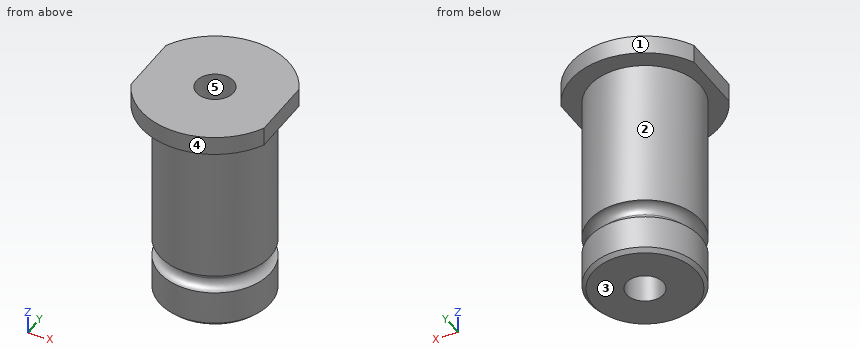
from build123d import *

# Parameters (mm, degrees)
F1_R     = 15
F2_DEPTH = 55
F3_R     = 20
F5_DEPTH = 5
F6_R     = 5
F7_DEPTH = 60.001
F9_DEPTH = 60.001
F10_R    = 2.5
F12_SIZE = 1


with BuildPart() as f2:
    # F1 (on Top) → F2 (new body)
    with BuildSketch(Plane.XY):
        Circle(F1_R)
    extrude(amount=F2_DEPTH)

    # F3 (on face) → F5 (join, through all)
    with BuildSketch(Plane.XY.offset(55)):
        Circle(F3_R)
    extrude(amount=F5_DEPTH)

    # F6 (on face) → F7 (cut, through all)
    with BuildSketch(Plane.XY.offset(60)):
        Circle(F6_R)
    extrude(amount=-F7_DEPTH, mode=Mode.SUBTRACT)

    # F8 (on face) → F9 (cut, through all)
    with BuildSketch(Plane.XY.offset(60)):
        with BuildLine():
            Line((-18, -8.7177978871), (-18, 0))
            Line((-18, 0), (-18, 8.7177978871))
            ThreePointArc((-18, 8.7177978871), (-20, 0), (-18, -8.7177978871))
        make_face()
        with BuildLine():
            Line((18, 8.7177978871), (18, 0))
            Line((18, 0), (18, -8.7177978871))
            ThreePointArc((18, -8.7177978871), (19.4935886896, -4.472135955), (20, 0))
            ThreePointArc((20, 0), (19.4935886896, 4.472135955), (18, 8.7177978871))
        make_face()
    extrude(amount=-F9_DEPTH, mode=Mode.SUBTRACT)

    # F10 (on Right) → F11 (revolve, cut)
    with BuildSketch(Plane.YZ):
        with Locations((-15, 12.5)):
            Circle(F10_R)
    revolve(axis=Axis((0, 0, 0), (0, 0, -1)), mode=Mode.SUBTRACT)

    # F12
    f12_edges = [f2.edges().sort_by_distance(p)[0] for p in [
        (-15, 0, 0),
    ]]
    chamfer(f12_edges, length=F12_SIZE)


solid = f2.part
Can you work these out from the model? Positions are in its coordinate system, mm. Face numbers are marked on the shaded views. A direction names the side the tool comes from. Round coordinates to 2 decimals unless told otherwise and drop trailing zeros. Loops run counter-clockwise (first coordinate to the right, second up) from the corner with the lowest first, then second, coordinate; pieces in that order, holes last. Notation, with made-up numbers: (-15, 78.25) - (-11, 78.25) arc R32 ccw to (-11, 111.25) - close; hole circle Ø7 at (-14.75, 73.5). An arc over 180 degrees is marked (long way). Write item = value, one per line. Start each with the question number.
(1) If we section it at C-C (z = 30.5): Please give me the cut outline in (x, y).
(2) If we section it at A-A (x = 0): Please give me the cut outline in (y, z).
(3) For the marked faces 1 and 2, which set-ups out of +Z, -Z, +X, -X, +Y, -Y let a thin tool reach every point of the face, with its end or its side?
(4) For P1, Ø10, axis at y = 13, z = 16.5, coming from the +X side; P2, Ø10, axis at y = -4, z = 6.5, coming from the +X side; P3, Ø10, axis at y = 11, z = 20, coming from the +X side, each with a flat end and sliding along its axis, tell me the tip position at first contact or that it passes through.
(5) If we mould it in two halves opening along X, with no side actions, what happens to the marked faces 3, 4 and 5? For each: released by +X, released by -X, zero draft, split by the parting line, or undercut.
(6) If I drill on probe 1 along Y at (x, z) = (0, 25); probe 2 along Z at (x, y) = (-15, -5); probe 3 along X at (y, z) = (-2.5, 51.5), over which ranges is the centre line in solid material (lowest first)? Write a range as [from, to].
(7) If we section it at B-B (y = 0): Please give me the cut outline in (x, z), and give its area (3 significant figures).
Ans:
q1.outline = circle Ø30 at (0, 0); hole circle Ø10 at (0, 0)
q2.outline = (-20, 55) - (-15, 55) - (-15, 15) arc R2.5 cw to (-15, 10) - (-15, 1) - (-14, 0) - (-5, 0) - (-5, 60) - (-20, 60) - close; (5, 0) - (14, 0) - (15, 1) - (15, 10) arc R2.5 cw to (15, 15) - (15, 55) - (20, 55) - (20, 60) - (5, 60) - close
q3.face_1 = +Z, -Z, +Y
q3.face_2 = -Z
q4.P1 = 12.69
q4.P2 = 15
q4.P3 = 13.75
q5.face_3 = zero draft
q5.face_4 = split by the parting line
q5.face_5 = undercut
q6.probe_1 = [-15, -5], [5, 15]
q6.probe_2 = [55, 60]
q6.probe_3 = [-14.79, -4.33], [4.33, 14.79]
q7.outline = (-18, 55) - (-15, 55) - (-15, 15) arc R2.5 cw to (-15, 10) - (-15, 1) - (-14, 0) - (-5, 0) - (-5, 60) - (-18, 60) - close; (5, 0) - (14, 0) - (15, 1) - (15, 10) arc R2.5 cw to (15, 15) - (15, 55) - (18, 55) - (18, 60) - (5, 60) - close
q7.area = 1,210 mm²
